Here's the drawing with two shaded views (mm, measured from the low corner). I have some questions. A direction names the side the tool comes from. Give positions to 0.01 mm unless a question says otherwise; leave off trailing zeros. Order: outer loops, then holes, each group sorted by start corner. A loop starts at its lowest first (then second) coordinate and runs counter-clockwise, first axis right, second up. Notation, with made-up numbers: (18, 57.5) - (29, 57.5) arc R21 ccw to (29, 96.5) - close; hole circle Ø10 at (80.25, -2). An arc over 180 degrees is marked (long way). Use one line per item in the form item = value. Start each with the question number.
1) Suppose I cut it at A-A, the plane x = 10. Write out the boundary of the cut face in (y, z).
2) For pin 1 (4 mm diameter, centred on x = 16.5, z = 2, fed in from +Y); pin 2 (0.8 mm diameter, centred on y = 0.5, z = 8.5, fed in from +X); pin 3 (0.5 mm diameter, centred on x = 9.5, y = 0.5, fed in from -Z); pin 4 (1.5 mm diameter, centred on x = 9.5, y = 0.5, fed in from -Z), each with a flat end and sliding along its axis, tell me the tip position at first contact or that it passes through.
3) We'd pull the mould along Y, two halves only. Please class the marked faces 1 and 2: released by +Y, released by -Y, zero draft, split by the parting line, or undercut.
4) Please list where these lines run through material, in increasing order: probe 1 along Z at (x, y) = (10, 2.5); probe 2 along Y at (x, z) = (15.25, 15.5); probe 3 along Y at (x, z) = (3.5, 4.25).
5) Suppose I cut it at D-D, the plane y = 2.55. Write out the boundary of the cut face in (x, z), and give its area (3 significant figures).
6) Suppose I cut it at C-C, the plane z = 9.5. Write out the boundary of the cut face in (x, y).
7) Suppose I cut it at B-B, the plane y = 0.7. Write out the boundary of the cut face in (x, z), and give its area (3 significant figures).
8) Which directions (+Z, -Z, +X, -X, +Y, -Y) give clear straight access to the entire face, cutting with the end or side of a thin tool? Please do the marked faces 3, 4 and 5.
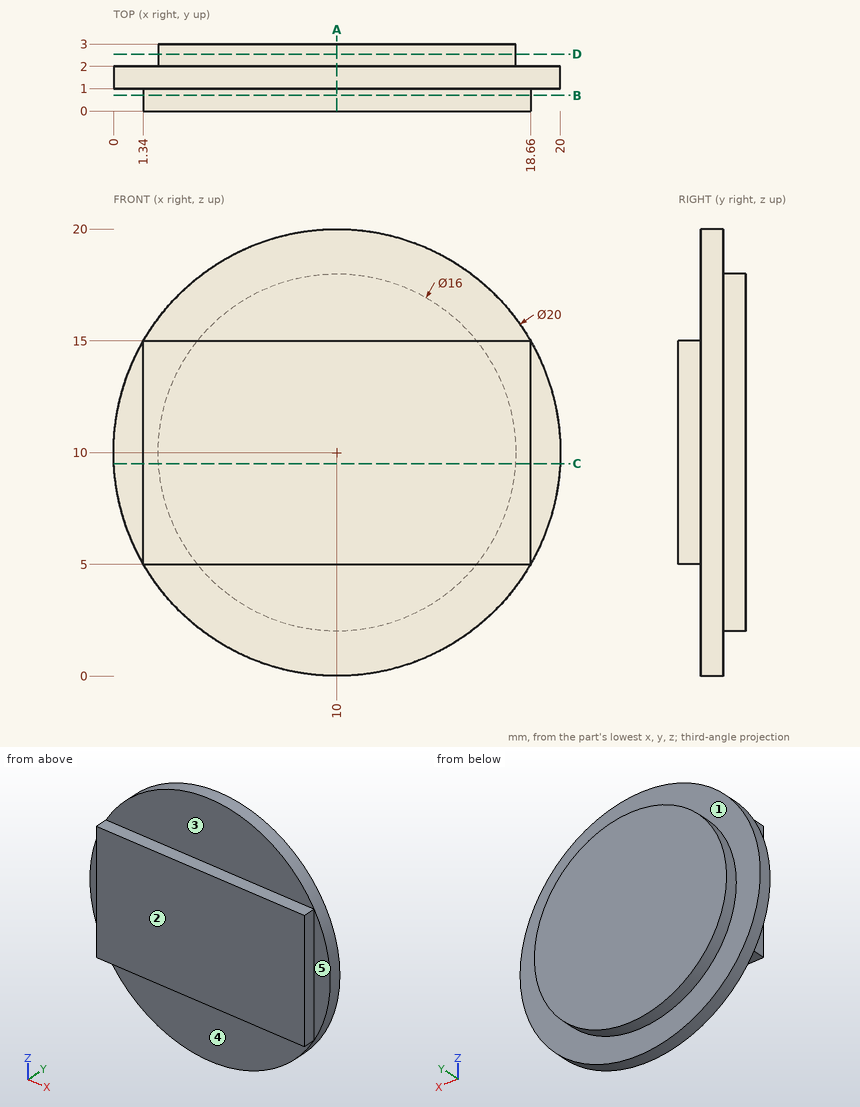
Result sheet:
q1.outline = (0, 5) - (1, 5) - (1, 0) - (2, 0) - (2, 2) - (3, 2) - (3, 18) - (2, 18) - (2, 20) - (1, 20) - (1, 15) - (0, 15) - close
q2.pin_1 = 2
q2.pin_2 = 18.66
q2.pin_3 = 5
q2.pin_4 = 0
q3.face_1 = released by +Y
q3.face_2 = released by -Y
q4.probe_1 = 2 to 18
q4.probe_2 = 1 to 3
q4.probe_3 = 1 to 2
q5.outline = circle Ø16 at (10, 10)
q5.area = 201 mm²
q6.outline = (0.01, 1) - (1.34, 1) - (1.34, 0) - (18.66, 0) - (18.66, 1) - (19.99, 1) - (19.99, 2) - (17.98, 2) - (17.98, 3) - (2.02, 3) - (2.02, 2) - (0.01, 2) - close
q7.outline = (1.34, 5) - (18.66, 5) - (18.66, 15) - (1.34, 15) - close
q7.area = 173 mm²
q8.face_3 = +Z, +X, -X, -Y
q8.face_4 = -Z, +X, -X, -Y
q8.face_5 = +Z, -Z, +X, -Y
